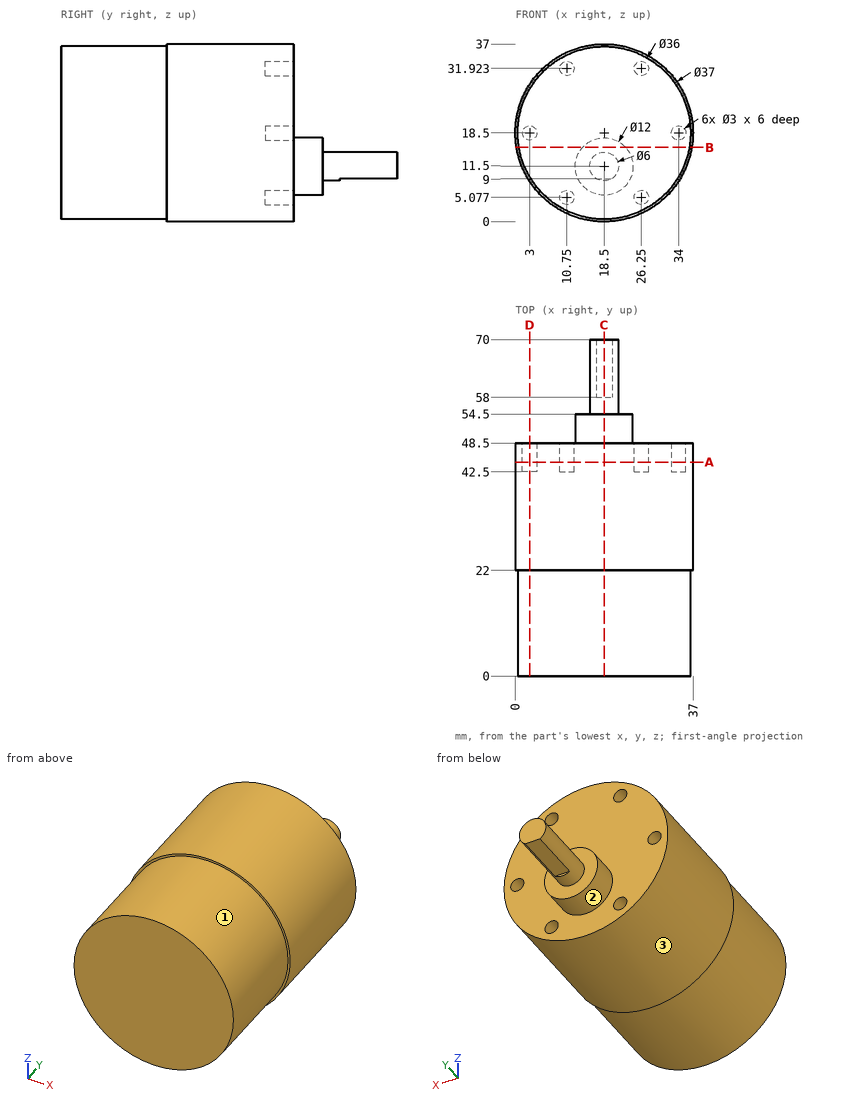
Here's the drawing with two shaded views (mm, measured from the low corner). I have some questions. A direction names the side the tool comes from. Round coordinates to 2 decimals unless told otherwise and drop trailing zeros. Write each loop counter-clockwise with the first axis right and the second up, starting at its lowest first coordinate (ties: lowest second). Pieces come first, ordered by that corner, then holes.
(1) Suppose I cut it at C-C on x = 18.5. Write out the boundary of the cut face in (y, z).
Findings below:
outline: (0, 0.5) - (22, 0.5) - (22, 0) - (48.5, 0) - (48.5, 5.5) - (54.5, 5.5) - (54.5, 8.5) - (58, 8.5) - (58, 9) - (70, 9) - (70, 14.5) - (54.5, 14.5) - (54.5, 17.5) - (48.5, 17.5) - (48.5, 37) - (22, 37) - (22, 36.5) - (0, 36.5) - close
(2) Suppose I cut it at D-D on x = 3. Write out the boundary of the cut face in (y, z), and give its area (3 significant figures).
Findings below:
outline: (0, 9.35) - (22, 9.35) - (22, 8.4) - (48.5, 8.4) - (48.5, 17) - (42.5, 17) - (42.5, 20) - (48.5, 20) - (48.5, 28.6) - (22, 28.6) - (22, 27.65) - (0, 27.65) - close
area: 920 mm2
(3) Suppose I cut it at B-B on z = 15.5. Write out the boundary of the cut face in (x, y) (1 decimal), and give its area (3 significant figures).
Findings below:
outline: (0.2, 22) - (0.8, 22) - (0.8, 0) - (36.2, 0) - (36.2, 22) - (36.8, 22) - (36.8, 48.5) - (23, 48.5) - (23, 54.5) - (14, 54.5) - (14, 48.5) - (0.2, 48.5) - close
area: 1,800 mm2
(4) For pin 1 (6 mm diameter, centred on y = 15.5, z = 24, fed in from -X) (1 decimal); pin 2 (1.5 mm diameter, centred on x = 3, z = 18.5, fed in from +Y); pin 3 (1 mm diameter, centred on x = 28, z = 16, fed in from +Y), each with a flat end and sliding along its axis, tell me the tip position at first contact or that it passes through.
Findings below:
pin 1: stops at x = 0.7
pin 2: stops at y = 42.5
pin 3: stops at y = 48.5
(5) Suppose I cut it at A-A on y = 44.5. State how many separate pieces and enclosed holes the cut face has, and give its area (3 significant figures).
Findings below:
separate pieces: 1
enclosed holes: 6
area: 1,030 mm2
(6) Which directions (+Z, -Z, +X, -X, +Y, -Y) give clear straight access to the entire face, cutting with the end or side of a thin tool? Please do the marked faces 1, 2 and 3.
Findings below:
face 1: -Y
face 2: +Y
face 3: +Y, -Y
(7) If I drill on probe 1 along Z at (x, y) = (26, 46) (1 decimal); probe 2 along Y at (x, z) = (17, 28); probe 3 along Z at (x, y) = (34, 44), over which ranges is the centre line in solid material (lowest first)?
Findings below:
probe 1: z = 1.6 to 3.6, 6.6 to 30.4, 33.4 to 35.4
probe 2: y = 0 to 48.5
probe 3: z = 8.4 to 17, 20 to 28.6
